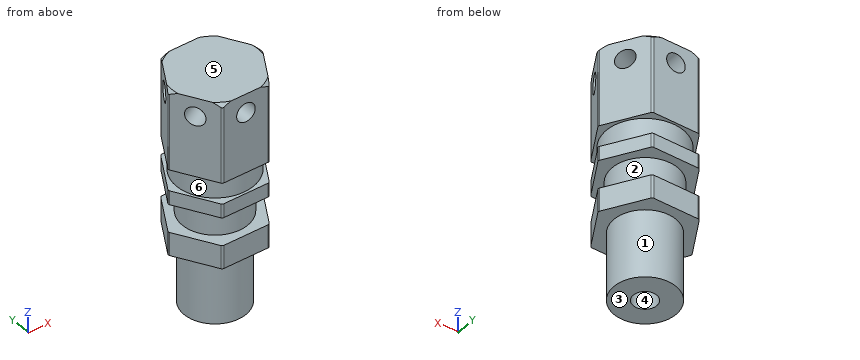
Autodesk Inventor part; units mm, degrees
ref_plane "YZ Plane" through (0, 0, 0) normal (1, 0, 0) x (0, 1, 0)
ref_plane "XZ Plane" through (0, 0, 0) normal (0, 1, 0) x (-1, 0, 0)
ref_plane "XY Plane" through (0, 0, 0) normal (0, 0, 1) x (1, 0, 0)
sketch "Sketch1" plane through (0, 0, 0) normal (0, 0, 1) x (1, 0, 0)
  line L0 (5.0518, 8.75) -> (10.1036, 0)
  line L1 (10.1036, 0) -> (5.0518, -8.75)
  line L2 (5.0518, -8.75) -> (-5.0518, -8.75)
  line L3 (-5.0518, -8.75) -> (-10.1036, 0)
  line L4 (-10.1036, 0) -> (-5.0518, 8.75)
  line L5 (-5.0518, 8.75) -> (5.0518, 8.75)
  point P0 (0, 0)
  point P1 (0, 0)
  dimension "d0" = 17.5
extrude "Extrusion1" add sketch "Sketch1" against normal blind 17
sketch "Sketch2" plane through (0, 0, -17) normal (0, 0, -1) x (-1, 0, 0)
  line L0 (-5.0518, 8.75) -> (5.0518, 8.75)
  line L1 (-10.1036, 0) -> (-5.0518, 8.75)
  line L2 (-5.0518, -8.75) -> (-10.1036, 0)
  line L3 (5.0518, -8.75) -> (-5.0518, -8.75)
  line L4 (10.1036, 0) -> (5.0518, -8.75)
  line L5 (5.0518, 8.75) -> (10.1036, 0)
  line L6 (-5.0518, 8.75) -> (5.0518, 8.75)
  circle A0 centre (0, 0) radius 8.25
  dimension "d3" = 16.5
extrude "Extrusion2" add sketch "Sketch2" along normal blind 4.5 contours A0
sketch "Sketch3" plane through (0, 0, -21.5) normal (0, 0, -1) x (-1, 0, 0)
  circle A0 centre (0, 0) radius 8.25
  line L0 (-5.0518, 8.75) -> (5.0518, 8.75)
  line L1 (-10.1036, 0) -> (-5.0518, 8.75)
  line L2 (-5.0518, -8.75) -> (-10.1036, 0)
  line L3 (5.0518, -8.75) -> (-5.0518, -8.75)
  line L4 (10.1036, 0) -> (5.0518, -8.75)
  line L5 (5.0518, 8.75) -> (10.1036, 0)
extrude "Extrusion3" add sketch "Sketch3" along normal blind 3 contours A0 | L0 L5 L4 L3 L2 L1
sketch "Sketch4" plane through (0, 0, -24.5) normal (0, 0, -1) x (-1, 0, 0)
  line L0 (5.0518, 8.75) -> (10.1036, 0)
  line L1 (-5.0518, 8.75) -> (5.0518, 8.75)
  line L2 (-10.1036, 0) -> (-5.0518, 8.75)
  line L3 (-5.0518, -8.75) -> (-10.1036, 0)
  line L4 (5.0518, -8.75) -> (-5.0518, -8.75)
  line L5 (10.1036, 0) -> (5.0518, -8.75)
  circle A0 centre (0, 0) radius 7
  dimension "d8" = 14
extrude "Extrusion4" add sketch "Sketch4" along normal blind 6 contours A0
sketch "Sketch5" plane through (0, 0, -30.5) normal (0, 0, -1) x (-1, 0, 0)
  circle A0 centre (0, 0) radius 7
  line L0 (5.0518, 8.75) -> (10.1036, 0)
  line L1 (-5.0518, 8.75) -> (5.0518, 8.75)
  line L2 (-10.1036, 0) -> (-5.0518, 8.75)
  line L3 (-5.0518, -8.75) -> (-10.1036, 0)
  line L4 (5.0518, -8.75) -> (-5.0518, -8.75)
  line L5 (10.1036, 0) -> (5.0518, -8.75)
extrude "Extrusion5" add sketch "Sketch5" along normal blind 5 contours A0 | L0 L5 L4 L3 L2 L1
sketch "Sketch6" plane through (0, 0, -35.5) normal (0, 0, -1) x (-1, 0, 0)
  line L0 (10.1036, 0) -> (5.0518, -8.75)
  line L1 (5.0518, 8.75) -> (10.1036, 0)
  line L2 (-5.0518, 8.75) -> (5.0518, 8.75)
  line L3 (-10.1036, 0) -> (-5.0518, 8.75)
  line L4 (-5.0518, -8.75) -> (-10.1036, 0)
  line L5 (5.0518, -8.75) -> (-5.0518, -8.75)
  circle A0 centre (0, 0) radius 6.625
  dimension "d13" = 13.25
extrude "Extrusion6" add sketch "Sketch6" along normal blind 14.5 contours A0
sketch "Sketch7" plane through (0, 0, -50) normal (0, 0, -1) x (-1, 0, 0)
  circle A0 centre (0, 0) radius 6.625
  circle A1 centre (0, 0) radius 2.5
  dimension "d16" = 5
extrude "Extrusion7" cut sketch "Sketch7" against normal blind 47.5 contours A1
sketch "Sketch8" plane through (-5.0518, 8.75, 0) normal (0, 1, 0) x (1, 0, 0)
  line L0 (10.1036, 17) -> (0, 17)
  line L1 (0, 0) -> (0, 17)
  line L2 (0, 0) -> (10.1036, 0)
  line L3 (10.1036, 0) -> (10.1036, 17)
  circle A0 centre (5.0518, 4) radius 2
  dimension "d19" = 4
  dimension "d20" = 4
extrude "Extrusion8" cut sketch "Sketch8" against normal blind 40.25 contours A0
pattern_circular "Circular Pattern1" count 3 over 360 about axis through (0, 0, -17) along (0, 0, -1) of "Extrusion8"
thread "Thread1"
fillet "Fillet1" radius 0.5 18 edges at (-5.0518, -8.75, -8.5) (5.0518, -8.75, -8.5) (10.1036, 0, -8.5) (5.0518, 8.75, -8.5) (-5.0518, 8.75, -8.5) (-10.1036, 0, -8.5) (-5.0518, -8.75, -23) (5.0518, -8.75, -23) (10.1036, 0, -23) (5.0518, 8.75, -23) (5.0518, 8.75, -33) (10.1036, 0, -33) (5.0518, -8.75, -33) (-5.0518, -8.75, -33) (-10.1036, 0, -23) (-5.0518, 8.75, -23) (-5.0518, 8.75, -33) (-10.1036, 0, -33)
sketch "Sketch10" plane through (0, 0, 0) normal (0, 1, 0) x (-1, 0, 0)
  line L0 (10.0263, 0) -> (10.0263, -17)
  line L1 (9.9593, 0) -> (5.1962, 0)
  line L2 (9.9593, -17) -> (9.9593, -17)
  line L3 (9.9593, -17) -> (9.9593, 0)
  line L4 (9.9593, 0) -> (9.9593, 0)
  line L5 (9.9593, 0) -> (9.9593, -17)
  ellipse E0 centre (7.5777, -4) end of major axis (7.5777, -2) minor radius 1
  line L6 (9.9593, 0) -> (9.9593, -17)
  line L7 (9.9593, 0) -> (5.1962, 0)
  line L8 (5.1962, -17) -> (5.1962, 0)
  line L9 (5.1962, -17) -> (9.9593, -17)
  line L10 (10.0263, -0.7071) -> (9.3192, 0)
  line L11 (9.3192, 0) -> (10.0263, 0)
  line L12 (10.0263, -0.7071) -> (10.0263, 0)
  line L13 (0, -20.4) -> (0, 3.4)
  dimension "d32" = 45
  dimension "d33" = 1
revolve "Revolution2" cut sketch "Sketch10" angle 360 about axis through (0, 0, -10) along (0, 0, 1) contours L0 L10 L3 L11 | L3 L10 L1
equation "\"d20\" = d19"
properties part number "fc18-055" material "Brass, Soft Yellow"
For this review, take the finished solid that the model builds, in its own axes (mm). Face numbers are marked on the shaded views. A direction names the side the tool comes from. Coordinates: 2 decimals unless noted, no trailing zeros. Loops run counter-clockwise (first coordinate to the right, second up) from the corner with the lowest first, then second, coordinate; pieces in that order, holes last. Notation, with made-up numbers: (-26.5, -24.75) - (19.5, -24.75) arc R15 cw to (19.5, -16.75) - close; hole circle Ø4 at (46.5, -21). An arc over 180 degrees is marked (long way). Return JSON: item names as keys, results as strings.
Item 1: For the marked faces 4, 5 and 6, list the 3-axis set-ups (+Z, -Z, +X, -X, +Y, -Y) from which the entire face can be reached by the end or side of a thin tool; tool diameter is ignored.
Determined:
{"face 4": "-Z", "face 5": "+Z, +X, -X, +Y, -Y", "face 6": "none"}
Item 2: Mouldability with a two-part tool opening along Z and no side actions: class the marked faces 1, 2 and 3 as pulls with the +Z half, pulls with the -Z half, needs draft (parallel to the pull), parting line crosses it, or undercut.
Determined:
{"face 1": "needs draft", "face 2": "undercut", "face 3": "pulls with the -Z half"}
Item 3: Take a section at A-A (z = -24). Give the boundary of the cut face in (x, y), then the cut area to 3 significant figures.
Determined:
{"outline": "(-9.96, -0.25) - (-5.2, -8.5) arc R0.5 ccw to (-4.76, -8.75) - (4.76, -8.75) arc R0.5 ccw to (5.2, -8.5) - (9.96, -0.25) arc R0.5 ccw to (9.96, 0.25) - (5.2, 8.5) arc R0.5 ccw to (4.76, 8.75) - (-4.76, 8.75) arc R0.5 ccw to (-5.2, 8.5) - (-9.96, 0.25) arc R0.5 ccw to start; hole circle Ø5 at (0, 0)", "area": "246 mm2"}
Item 4: For line 1 (Z direction, x = -5.25, y = 8); line 2 (Z direction, x = 2.75, y = 8); line 3 (Y direction, x = 0, z = -26), list the stretches that pass through material, from the lowest coordinate up.
Determined:
{"line 1": "z = -35.5 to -30.5, -24.5 to -21.5, -17 to -0.25", "line 2": "z = -35.5 to -30.5, -24.5 to -21.5, -17 to 0", "line 3": "y = -7 to -2.5, 2.5 to 7"}
Item 5: Insertion check: pin 1 (12 mm diameter, centred on x = -0.5, z = -42.5, fed in from +Y) (3 decimals); pin 2 (1 mm diameter, centred on y = 3.5, z = -15.5, fed in from -X); pin 3 (1 mm diameter, centred on x = -6, z = -6, fed in from +Y). Each pin has a flat end and moves straight along its axis. Give the tip position at first contact, or say it passes through.
Determined:
{"pin 1": "stops at y = 6.625", "pin 2": "stops at x = -8.37", "pin 3": "stops at y = 7.97"}
Item 6: Take a section at B-B (z = -4). State how many separate pieces and enclosed holes the cut face has, then the cut area to 3 significant figures.
Determined:
{"separate pieces": "6", "enclosed holes": "0", "area": "96.7 mm2"}
Item 7: Take a section at C-C (z = -44). Give the boundary of the cut face in (x, y) (3 decimals).
Determined:
{"outline": "circle Ø13.25 at (0, 0); hole circle Ø5 at (0, 0)"}
